The model under review builds one solid part; all positions refer to its coordinate system, in mm. Face numbers are marked on the shaded views. A direction names the side the tool comes from. Give positions to 0.01 mm unless a question says otherwise; leave off trailing zeros. Order: outer loops, then holes, each group sorted by start corner. A loop starts at its lowest first (then second) coordinate and runs counter-clockwise, first axis right, second up.
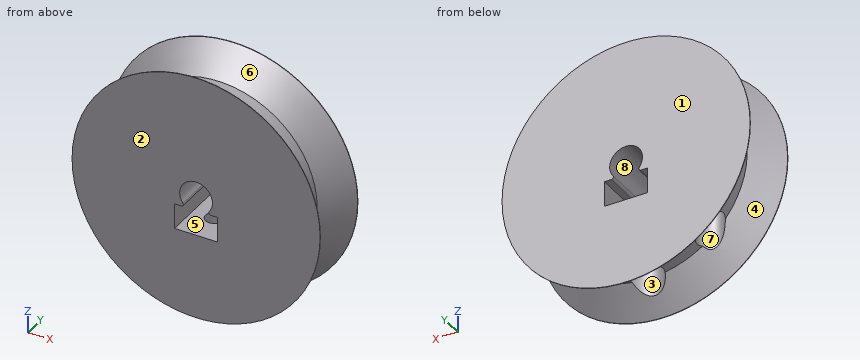
```python
from build123d import *

# Parameters (mm, degrees)
CUT_EXTRUDE2_DEPTH      = 13.7
SKETCH9_W               = 8.382
SKETCH9_H               = 4.953
CUT_EXTRUDE3_DEPTH      = 13.7
FILLET2_R               = 0.396875
SKETCH14_W              = 1.7272
SKETCH14_H              = 21.5665
SKETCH15_R              = 3.429
CUT_EXTRUDE4_DEPTH      = 5.9800001
CUT_EXTRUDE4_DEPTH_BACK = 6.096
CUT_EXTRUDE6_START      = -19.15
SKETCH16_R              = 1.27
CUT_EXTRUDE6_DEPTH      = 25.1300001
CUT_EXTRUDE7_START      = -19.15
SKETCH16_3_R            = 2.54
CUT_EXTRUDE7_DEPTH      = 25.1300001


with BuildPart() as part:
    # Sketch7 → Revolve1 (revolve)
    with BuildSketch(Plane.XY):
        Polygon((0, 0), (24.13, 0), (24.13, 0.1), (19.15, 5.08), (19.15, 7.62), (24.13, 12.6), (24.13, 12.7), (0, 12.7), align=None)
    revolve(axis=Axis((0, 12.7, 0), (0, -1, 0)))

    # Sketch8 → Cut-Extrude2 (cut, through all)
    with BuildSketch(Plane(origin=(0, 12.7, 0), x_dir=(1, 0, 0), z_dir=(0, 1, 0))):
        with BuildLine():
            Line((-1.899409908, 2.5635), (1.899409908, 2.5635))
            ThreePointArc((1.899409908, 2.5635), (0, -3.1905), (-1.899409908, 2.5635))
        make_face()
    extrude(amount=-CUT_EXTRUDE2_DEPTH, mode=Mode.SUBTRACT)

    # Sketch9 → Cut-Extrude3 (cut, through all)
    with BuildSketch(Plane(origin=(0, 12.7, 0), x_dir=(1, 0, 0), z_dir=(0, 1, 0))):
        with Locations((0, 5.04)):
            Rectangle(SKETCH9_W, SKETCH9_H)
    extrude(amount=-CUT_EXTRUDE3_DEPTH, mode=Mode.SUBTRACT)

    # Fillet2
    fillet2_edges = [part.edges().sort_by_distance(p)[0] for p in [
        (1.899409908, 6.35, -2.5635),
        (-1.899409908, 6.35, -2.5635),
    ]]
    fillet(fillet2_edges, radius=FILLET2_R)

    # Sketch14 → #8-32 Tapped Hole1 (revolve, cut)
    with BuildSketch(Plane(origin=(0, 6.153258969, -2.5635), x_dir=(0, -1, 0), z_dir=(1, 0, 0))):
        with Locations((0.8636, 10.78325)):
            Rectangle(SKETCH14_W, SKETCH14_H)
    revolve(axis=Axis((0, 6.153258969, 3.7865), (0, 0, -1)), mode=Mode.SUBTRACT)

    # Sketch15 → Cut-Extrude4 (cut, two sides)
    with BuildSketch(Plane(origin=(0, 0, -19.15), x_dir=(-1, 0, 0), z_dir=(0, 0, -1))) as cut_extrude4_sk:
        with Locations((0, 6.35)):
            Circle(SKETCH15_R)
    extrude(amount=CUT_EXTRUDE4_DEPTH, mode=Mode.SUBTRACT)
    extrude(cut_extrude4_sk.sketch, amount=-CUT_EXTRUDE4_DEPTH_BACK, mode=Mode.SUBTRACT)

    # Sketch16 → Cut-Extrude6 (cut, through all)
    with BuildSketch(Plane(origin=(0, 0, -19.15), x_dir=(-1, 0, 0), z_dir=(0, 0, -1)).offset(CUT_EXTRUDE6_START)):
        with Locations((12.7, 6.35)):
            Circle(SKETCH16_R)
    extrude(amount=-CUT_EXTRUDE6_DEPTH, mode=Mode.SUBTRACT)

    # Sketch16<3> → Cut-Extrude7 (cut, through all)
    with BuildSketch(Plane(origin=(0, 0, -19.15), x_dir=(-1, 0, 0), z_dir=(0, 0, -1)).offset(CUT_EXTRUDE7_START)):
        with Locations((12.7, 6.35)):
            Circle(SKETCH16_3_R)
    extrude(amount=CUT_EXTRUDE7_DEPTH, mode=Mode.SUBTRACT)


solid = part.part
```
Item 1: For line 1 (X direction, y = 4.5, z = -5); line 2 (Y direction, x = 0, z = -9.5); line 3 (Y direction, x = -12.7, z = 7.75), list the stretches that pass through material, from the lowest coordinate up.
Values found:
line 1: x = -19.09 to -14.44, -10.96 to -4.19, 4.19 to 19.09
line 2: y = 0 to 4.43, 7.88 to 12.7
line 3: y = 0 to 5.08, 7.62 to 12.7
Item 2: Take a section at C-C (y = 6.35). Give the boundary of the cut face in (x, z).
Values found:
outline: (-15.24, -11.6) - (-15.24, 0) - (-13.97, 0) - (-13.97, 13.1) arc R19.15 ccw to start; (-11.43, 0) - (-10.16, 0) - (-10.16, -16.23) arc R19.15 ccw to (-3.43, -18.84) - (-3.43, -13.05) - (-1.72, -13.05) - (-1.72, -7.52) - (-4.19, -7.52) - (-4.19, -2.56) - (-2.86, -2.56) arc R0.4 ccw to (-2.54, -1.93) arc R3.19 cw (long way) to (2.54, -1.93) arc R0.4 ccw to (2.86, -2.56) - (4.19, -2.56) - (4.19, -7.52) - (1.72, -7.52) - (1.72, -13.05) - (3.43, -13.05) - (3.43, -18.84) arc R19.15 ccw (long way) to (-11.43, 15.36) - close
Item 3: For the marked faces 1, 2, 3, 4 and 5, list the 3-axis set-ups (+Z, -Z, +X, -X, +Y, -Y) from which the entire face can be reached by the end or side of a thin tool; tool diameter is ignored.
Values found:
face 1: +Z, -Z, +X, -X, +Y
face 2: +Z, -Z, +X, -X, -Y
face 3: -Z
face 4: none
face 5: +Y, -Y
Item 4: Take a section at B-B (y = 11). Give the boundary of the cut face in (x, z), and give its area (3 significant figures).
Values found:
outline: circle Ø45.06 at (0, 0); hole (-4.19, -7.52) - (4.19, -7.52) - (4.19, -2.56) - (2.86, -2.56) arc R0.4 cw to (2.54, -1.93) arc R3.19 ccw (long way) to (-2.54, -1.93) arc R0.4 cw to (-2.86, -2.56) - (-4.19, -2.56) - close
area: 1,520 mm2
Item 5: Take a section at A-A (x = 0). Give the boundary of the cut face in (y, z), and give its area (3 significant figures).
Values found:
outline: (0, -24.13) - (0.1, -24.13) - (2.92, -21.31) - (2.92, -13.05) - (4.43, -13.05) - (4.43, -7.52) - (0, -7.52) - close; (0, 3.19) - (12.7, 3.19) - (12.7, 24.13) - (12.6, 24.13) - (7.62, 19.15) - (5.08, 19.15) - (0.1, 24.13) - (0, 24.13) - close; (7.88, -13.05) - (9.78, -13.05) - (9.78, -21.31) - (12.6, -24.13) - (12.7, -24.13) - (12.7, -7.52) - (7.88, -7.52) - close
area: 336 mm2
Item 6: Take a section at D-D (z = -4). Give the number of separate pieces and of enclosed holes in the cut face, and give its area (3 significant figures).
Values found:
separate pieces: 2
enclosed holes: 1
area: 402 mm2
Item 7: Clearance check with flat-ended pins moving along their axes: pin 1 Ø6 at (x, y) = (0, 6.35) entering from -Z; pin 2 Ø5.5 at (y, z) = (3.5, -4) entering from -X; pin 3 Ø1.5 at (x, y) = (-3.5, 4) entering from -Z; pin 4 Ø1.5 at (x, z) = (13, -14.5) entering from -Y. State where each tip first meets the part, or that it passes through.
Values found:
pin 1: stops at z = -13.05
pin 2: stops at x = -23.17
pin 3: stops at z = -20.7
pin 4: stops at y = 0
Item 8: Draft analysis for pull direction Z (two halves, no side actions). For the marked faces 6, 7 and 8, state which applies: released by +Z, released by -Z, zero draft, split by the parting line, or undercut.
Values found:
face 6: split by the parting line
face 7: zero draft
face 8: undercut
